from build123d import *

# Parameters (mm, degrees)
SKETCH1_W           = 139
SKETCH1_H           = 160
BOSS_EXTRUDE1_DEPTH = 5
SKETCH2_W           = 16
SKETCH2_H           = 16
CUT_EXTRUDE1_DEPTH  = 5
SKETCH3_R           = 2.15
CUT_EXTRUDE2_DEPTH  = 5
SKETCH4_R           = 2.15
CUT_EXTRUDE3_DEPTH  = 5
LPATTERN1_COUNT     = 4
LPATTERN1_PITCH     = 35
SKETCH5_R           = 2.15
CUT_EXTRUDE4_DEPTH  = 5
SKETCH6_W           = 109
SKETCH6_H           = 15
BOSS_EXTRUDE2_DEPTH = 5
SKETCH7_W           = 55
SKETCH7_H           = 104
CUT_EXTRUDE5_DEPTH  = 5
SKETCH8_R           = 2.15
CUT_EXTRUDE6_DEPTH  = 5


with BuildPart() as part:
    # Sketch1 → Boss-Extrude1 (new body)
    with BuildSketch(Plane.XY):
        with Locations((69.5, 80)):
            Rectangle(SKETCH1_W, SKETCH1_H)
    extrude(amount=BOSS_EXTRUDE1_DEPTH)

    # Sketch2 → Cut-Extrude1 (cut)
    with BuildSketch(Plane.XY.offset(5)):
        with Locations((131, 152)):
            Rectangle(SKETCH2_W, SKETCH2_H)
        with Locations((8, 152)):
            Rectangle(SKETCH2_W, SKETCH2_H)
    extrude(amount=-CUT_EXTRUDE1_DEPTH, mode=Mode.SUBTRACT)

    # Sketch3 → Cut-Extrude2 (cut)
    with BuildSketch(Plane.XY.offset(5)):
        with Locations((69.5, 152.5)):
            Circle(SKETCH3_R)
        with Locations((44.5, 152.5)):
            Circle(SKETCH3_R)
        with Locations(Location((94.5, 152.5, 0), (0, 0, 180))):
            Circle(SKETCH3_R)
    extrude(amount=-CUT_EXTRUDE2_DEPTH, mode=Mode.SUBTRACT)

    # Sketch4 → Cut-Extrude3 (cut)
    with BuildSketch(Plane.XY.offset(5)):
        with Locations((131.5, 129)):
            Circle(SKETCH4_R)
        with Locations(Location((7.5, 129, 0), (0, 0, 180))):
            Circle(SKETCH4_R)
    cut_extrude3 = extrude(amount=-CUT_EXTRUDE3_DEPTH, mode=Mode.SUBTRACT)

    # LPattern1: Cut-Extrude3 ×4
    with Locations(*[(0, -i * LPATTERN1_PITCH, 0) for i in range(1, LPATTERN1_COUNT)]):
        add(cut_extrude3, mode=Mode.SUBTRACT)

    # Sketch5 → Cut-Extrude4 (cut)
    with BuildSketch(Plane.XY.offset(5)):
        with Locations((117, 112)):
            Circle(SKETCH5_R)
        with Locations((117, 87)):
            Circle(SKETCH5_R)
        with Locations(Location((22, 87, 0), (0, 0, 180))):
            Circle(SKETCH5_R)
        with Locations(Location((22, 112, 0), (0, 0, 180))):
            Circle(SKETCH5_R)
    extrude(amount=-CUT_EXTRUDE4_DEPTH, mode=Mode.SUBTRACT)

    # Sketch6 → Boss-Extrude2 (add)
    with BuildSketch(Plane(origin=(0, 0, 0), x_dir=(-1, 0, 0), z_dir=(0, 0, -1))):
        with Locations((-69.5, -7.5)):
            Rectangle(SKETCH6_W, SKETCH6_H)
    extrude(amount=-BOSS_EXTRUDE2_DEPTH)

    # Sketch7 → Cut-Extrude5 (cut)
    with BuildSketch(Plane.XY.offset(5)):
        with Locations((69.5, 47)):
            Rectangle(SKETCH7_W, SKETCH7_H)
    extrude(amount=-CUT_EXTRUDE5_DEPTH, mode=Mode.SUBTRACT)

    # Sketch8 → Cut-Extrude6 (cut)
    with BuildSketch(Plane.XY.offset(5)):
        with Locations((102, 5)):
            Circle(SKETCH8_R)
        with Locations((102, 120)):
            Circle(SKETCH8_R)
        with Locations(Location((37, 120, 0), (0, 0, 180))):
            Circle(SKETCH8_R)
        with Locations(Location((37, 5, 0), (0, 0, 180))):
            Circle(SKETCH8_R)
    extrude(amount=-CUT_EXTRUDE6_DEPTH, mode=Mode.SUBTRACT)


solid = part.part
Could you check a few things on this model? Use its own coordinates, in mm. A direction names the side the tool comes from. Coordinates: 2 decimals unless noted, no trailing zeros. Loops run counter-clockwise (first coordinate to the right, second up) from the corner with the lowest first, then second, coordinate; pieces in that order, holes last.
1. We'd pull the mould along X, two halves only. Please class faces 1 (the face through (70, -15, 2)), 2 (the face through (132.49, 127.09, 2.54)), 3 (the face through (15, -8, 2)), 4 (the face through (133.486, 93.177, 2.535)): released by +X, released by -X, zero draft, split by the parting line, or undercut.
2. For faces 5 (the face through (131, 0, 2)), 6 (the face through (99, 74, 0)), 7 (the face through (69, -5, 3)), 8 (the face through (8, 144, 3)), 9 (the face through (0, 71, 2)), which set-ups out of +Z, -Z, +X, -X, +Y, -Y let a thin tool reach every point of the face, with its end or its side?
3. Imagine slicing it at D-D (y = 120). Please give me the cut outline in (x, z), and give its area (3 significant figures).
4. Imagine slicing it at C-C (y = 24). Please give me the cut outline in (x, z), and give its area (3 significant figures).
5. Imagine slicing it at B-B (x = 102). Please give me the cut outline in (y, z).
6. For P1, Ø2.5, axis at y = 153.5, z = 1.5, coming from the -X side; P2, Ø2.5, axis at x = 134, z = 3, coming from the -Y side; P3, Ø2.5, axis at y = -6, z = 2, coming from the -X side, each with a flat end and sliding along its axis, tell me the tip position at first contact or that it passes through.
7. I need wall thicknesses on L1, parallel to Y at x = 102, z = 3.15; L2, parallel to X at y = 24, z = 2.7; L3, parallel to Y at x = 22, z = 1.15. Which ranges of each line are inside material? Lowest first, please.
8. Imagine slicing it at A-A (y = 83). Please give me the cut outline in (x, z), and give its area (3 significant figures).
Computed values:
1. face 1: zero draft
1. face 2: undercut
1. face 3: released by -X
1. face 4: undercut
2. face 5: +Z, -Z, +X, -Y
2. face 6: -Z, +X, -X, +Y, -Y
2. face 7: +Z, -Z
2. face 8: +Z, -Z, -X, +Y
2. face 9: +Z, -Z, -X, +Y, -Y
3. outline: (0, 0) - (34.85, 0) - (34.85, 5) - (0, 5) - close; (39.15, 0) - (99.85, 0) - (99.85, 5) - (39.15, 5) - close; (104.15, 0) - (139, 0) - (139, 5) - (104.15, 5) - close
3. area: 652 mm2
4. outline: (0, 0) - (5.35, 0) - (5.35, 5) - (0, 5) - close; (9.65, 0) - (42, 0) - (42, 5) - (9.65, 5) - close; (97, 0) - (129.35, 0) - (129.35, 5) - (97, 5) - close; (133.65, 0) - (139, 0) - (139, 5) - (133.65, 5) - close
4. area: 377 mm2
5. outline: (-15, 0) - (2.85, 0) - (2.85, 5) - (-15, 5) - close; (7.15, 0) - (117.85, 0) - (117.85, 5) - (7.15, 5) - close; (122.15, 0) - (160, 0) - (160, 5) - (122.15, 5) - close
6. P1: stops at x = 16
6. P2: stops at y = 0
6. P3: stops at x = 15
7. L1: y = -15 to 2.85, 7.15 to 117.85, 122.15 to 160
7. L2: x = 0 to 5.35, 9.65 to 42, 97 to 129.35, 133.65 to 139
7. L3: y = -15 to 84.85, 89.15 to 109.85, 114.15 to 160
8. outline: (0, 0) - (42, 0) - (42, 5) - (0, 5) - close; (97, 0) - (139, 0) - (139, 5) - (97, 5) - close
8. area: 420 mm2
